```python
from build123d import *

# Parameters (mm, degrees)
BOSS_EXTRUDE1_DEPTH = 10
BOSS_EXTRUDE2_DEPTH = 50


with BuildPart() as part:
    # Sketch1 → Boss-Extrude1 (new body)
    with BuildSketch(Plane.XY):
        Polygon((0, 150), (50, 150), (50, 50), (100, 50), (100, 0), (0, 0), align=None)
    extrude(amount=BOSS_EXTRUDE1_DEPTH)

    # Sketch2 → Boss-Extrude2 (add)
    with BuildSketch(Plane.XY.offset(10)):
        Polygon((40, 150), (40, 40), (100, 40), (100, 50), (50, 50), (50, 150), align=None)
    extrude(amount=BOSS_EXTRUDE2_DEPTH)

    # Sketch3 → CBORE for #10 Binding Head Machine Screw1 (revolve, cut)
    with BuildSketch(Plane(origin=(25.416829558, 24.242970072, 10), x_dir=(0, -1, 0), z_dir=(1, 0, 0))):
        Polygon((0, 0), (0, 10), (2.5527, 10), (2.5527, 3.1242), (5.55625, 3.1242), (5.55625, 0.635), (6.19125, 0), align=None)
    revolve(axis=Axis((25.416829558, 24.242970072, 16.35), (0, 0, -1)), mode=Mode.SUBTRACT)


solid = part.part
```
Geometry: final body of the model. Coordinates: model frame, mm. A direction names the side the tool comes from. Round coordinates to 2 decimals unless told otherwise and drop trailing zeros. Order: outer loops, then holes, each group sorted by start corner. A loop starts at its lowest first (then second) coordinate and runs counter-clockwise, first axis right, second up. Notation, with made-up numbers: (50.25, 83) - (99.25, 83) arc R11 ccw to (99.25, 94) - close; hole circle Ø11 at (41, 26.5). An arc over 180 degrees is marked (long way). Use CSV: the item, a comma, the result in double quotes. Start each with the question number.
Q1. Section query C-C (x = 12). Return loops of the section in (y, z), and give its area (3 significant figures).
Q2. Section query B-B (x = 60). Return loops of the section in (y, z), and give its area (3 significant figures).
Q3. First-contact query: pin 1 (12 mm diameter, centred on x = 24.5, y = 25, fed in from +Z); pin 2 (12 mm diameter, centred on x = 75.5, z = 29, fed in from +Y); pin 3 (25 mm diameter, centred on y = 102.5, z = 40.5, fed in from -X). Flat tips, straight axial feed; report the tip coordinate or a pass-through.
Q4. Material intervals for line 1 along Y through (x, z) = (55.5, 5); line 2 along Y through (x, z) = (91.5, 34.5), sorted ascending. Write a range as from..to.
Q5. Access query for faces 4 (the face through (20.73, 21.26, 8.14)), 5 (the face through (51, 0, 5)), 6 (the face through (75, 50, 30)), 7 (the face through (0, 74, 5)), 8 (the face through (70, 40, 35)). Directions: +Z, -Z, +X, -X, +Y, -Y. A direction counts if a zero-diameter tool reaches every point of the face in a straight line with its end or side. Return the directions, or none.
Q6. Mould query, pull axis X, two halves, no side actions, for faces 1 (the face through (27, 27, 6.876)), 2 (the face through (40, 96, 35)), 3 (the face through (48, 87, 60)). Classes: +X half, -X half, draft (parallel to the pull), parting line (faces both ways), or undercut.
Q7. Section query A-A (z = 13). Return loops of the section in (x, y).
Result set:
1,outline,"(0, 0) - (150, 0) - (150, 10) - (0, 10) - close"
1,area,"1,500 mm2"
2,outline,"(0, 0) - (50, 0) - (50, 60) - (40, 60) - (40, 10) - (0, 10) - close"
2,area,"1,000 mm2"
3,pin 1,"stops at z = 10"
3,pin 2,"stops at y = 50"
3,pin 3,"stops at x = 40"
4,line 1,"y = 0..50"
4,line 2,"y = 40..50"
5,face 4,"+Z"
5,face 5,"+Z, -Z, +X, -X, -Y"
5,face 6,"+Z, -Z, +X, +Y"
5,face 7,"+Z, -Z, -X, +Y, -Y"
5,face 8,"+Z, +X, -X, -Y"
6,face 1,"undercut"
6,face 2,"-X half"
6,face 3,"draft"
7,outline,"(40, 40) - (100, 40) - (100, 50) - (50, 50) - (50, 150) - (40, 150) - close"
